from build123d import *

# Parameters (mm, degrees)
SKETCH_1_R          = 36.5
SKETCH_1_R_2        = 28
EXTRUDE_1_DEPTH     = 5.5
SKETCH_2_R          = 31.1
CUT_EXTRUDE_1_DEPTH = 3.3
CUT_EXTRUDE_2_REACH = 53.911
SKETCH_3_R          = 1.55
SKETCH_4_R          = 1.55
CUT_EXTRUDE_3_DEPTH = 3.2


with BuildPart() as part:
    # 草图1 → 凸台-拉伸1 (new body)
    with BuildSketch(Plane(origin=(0, 0, 0), x_dir=(0, 0, -1), z_dir=(1, 0, 0))):
        Circle(SKETCH_1_R)
        Circle(SKETCH_1_R_2, mode=Mode.SUBTRACT)
    extrude(amount=EXTRUDE_1_DEPTH)

    # 草图2 → 切除-拉伸1 (cut)
    with BuildSketch(Plane.ZY):
        Circle(SKETCH_2_R)
    extrude(amount=-CUT_EXTRUDE_1_DEPTH, mode=Mode.SUBTRACT)

    # 草图3 → 切除-拉伸2 (cut, up to next)
    with BuildSketch(Plane(origin=(5.5, 0, 0), x_dir=(0, 0, -1), z_dir=(1, 0, 0)), mode=Mode.PRIVATE) as cut_extrude_2_sk1:
        with Locations((32.9, 0)):
            Circle(SKETCH_3_R)
    cut_extrude_2_tool1 = extrude(cut_extrude_2_sk1.sketch, amount=-CUT_EXTRUDE_2_REACH, mode=Mode.PRIVATE) & part.part
    # 草图3 → 切除-拉伸2 (cut, up to next)
    with BuildSketch(Plane(origin=(5.5, 0, 0), x_dir=(0, 0, -1), z_dir=(1, 0, 0)), mode=Mode.PRIVATE) as cut_extrude_2_sk2:
        with Locations((23.263813101, -23.263813101)):
            Circle(SKETCH_3_R)
    cut_extrude_2_tool2 = extrude(cut_extrude_2_sk2.sketch, amount=-CUT_EXTRUDE_2_REACH, mode=Mode.PRIVATE) & part.part
    # 草图3 → 切除-拉伸2 (cut, up to next)
    with BuildSketch(Plane(origin=(5.5, 0, 0), x_dir=(0, 0, -1), z_dir=(1, 0, 0)), mode=Mode.PRIVATE) as cut_extrude_2_sk3:
        with Locations((0, -32.9)):
            Circle(SKETCH_3_R)
    cut_extrude_2_tool3 = extrude(cut_extrude_2_sk3.sketch, amount=-CUT_EXTRUDE_2_REACH, mode=Mode.PRIVATE) & part.part
    # 草图3 → 切除-拉伸2 (cut, up to next)
    with BuildSketch(Plane(origin=(5.5, 0, 0), x_dir=(0, 0, -1), z_dir=(1, 0, 0)), mode=Mode.PRIVATE) as cut_extrude_2_sk4:
        with Locations((-23.263813101, -23.263813101)):
            Circle(SKETCH_3_R)
    cut_extrude_2_tool4 = extrude(cut_extrude_2_sk4.sketch, amount=-CUT_EXTRUDE_2_REACH, mode=Mode.PRIVATE) & part.part
    # 草图3 → 切除-拉伸2 (cut, up to next)
    with BuildSketch(Plane(origin=(5.5, 0, 0), x_dir=(0, 0, -1), z_dir=(1, 0, 0)), mode=Mode.PRIVATE) as cut_extrude_2_sk5:
        with Locations((-32.9, 0)):
            Circle(SKETCH_3_R)
    cut_extrude_2_tool5 = extrude(cut_extrude_2_sk5.sketch, amount=-CUT_EXTRUDE_2_REACH, mode=Mode.PRIVATE) & part.part
    # 草图3 → 切除-拉伸2 (cut, up to next)
    with BuildSketch(Plane(origin=(5.5, 0, 0), x_dir=(0, 0, -1), z_dir=(1, 0, 0)), mode=Mode.PRIVATE) as cut_extrude_2_sk6:
        with Locations((-23.263813101, 23.263813101)):
            Circle(SKETCH_3_R)
    cut_extrude_2_tool6 = extrude(cut_extrude_2_sk6.sketch, amount=-CUT_EXTRUDE_2_REACH, mode=Mode.PRIVATE) & part.part
    # 草图3 → 切除-拉伸2 (cut, up to next)
    with BuildSketch(Plane(origin=(5.5, 0, 0), x_dir=(0, 0, -1), z_dir=(1, 0, 0)), mode=Mode.PRIVATE) as cut_extrude_2_sk7:
        with Locations((0, 32.9)):
            Circle(SKETCH_3_R)
    cut_extrude_2_tool7 = extrude(cut_extrude_2_sk7.sketch, amount=-CUT_EXTRUDE_2_REACH, mode=Mode.PRIVATE) & part.part
    # 草图3 → 切除-拉伸2 (cut, up to next)
    with BuildSketch(Plane(origin=(5.5, 0, 0), x_dir=(0, 0, -1), z_dir=(1, 0, 0)), mode=Mode.PRIVATE) as cut_extrude_2_sk8:
        with Locations((23.263813101, 23.263813101)):
            Circle(SKETCH_3_R)
    cut_extrude_2_tool8 = extrude(cut_extrude_2_sk8.sketch, amount=-CUT_EXTRUDE_2_REACH, mode=Mode.PRIVATE) & part.part
    add(cut_extrude_2_tool1.solids().sort_by_distance((5.5, 0, -32.9))[0], mode=Mode.SUBTRACT)
    add(cut_extrude_2_tool2.solids().sort_by_distance((5.5, -23.263813, -23.263813))[0], mode=Mode.SUBTRACT)
    add(cut_extrude_2_tool3.solids().sort_by_distance((5.5, -32.9, 0))[0], mode=Mode.SUBTRACT)
    add(cut_extrude_2_tool4.solids().sort_by_distance((5.5, -23.263813, 23.263813))[0], mode=Mode.SUBTRACT)
    add(cut_extrude_2_tool5.solids().sort_by_distance((5.5, 0, 32.9))[0], mode=Mode.SUBTRACT)
    add(cut_extrude_2_tool6.solids().sort_by_distance((5.5, 23.263813, 23.263813))[0], mode=Mode.SUBTRACT)
    add(cut_extrude_2_tool7.solids().sort_by_distance((5.5, 32.9, 0))[0], mode=Mode.SUBTRACT)
    add(cut_extrude_2_tool8.solids().sort_by_distance((5.5, 23.263813, -23.263813))[0], mode=Mode.SUBTRACT)

    # 草图4 → 切除-拉伸3 (cut)
    # profile 1 of 8: a face of its own
    with BuildSketch(Plane(origin=(5.5, 0, 0), x_dir=(0, 0, -1), z_dir=(1, 0, 0))):
        with BuildLine():
            Line((-32.656757596, 2.889780811), (-36.359328813, 3.20143847))
            ThreePointArc((-36.359328813, 3.20143847), (-36.5, 0), (-36.359328813, -3.20143847))
            Line((-36.359328813, -3.20143847), (-32.656757596, -2.889780811))
            ThreePointArc((-32.656757596, -2.889780811), (-30, 0), (-32.656757596, 2.889780811))
        make_face()
        with Locations((-32.9, 0)):
            Circle(SKETCH_4_R, mode=Mode.SUBTRACT)
    # profile 2 of 8: a face of its own
    with BuildSketch(Plane(origin=(5.5, 0, 0), x_dir=(0, 0, -1), z_dir=(1, 0, 0))):
        with BuildLine():
            Line((2.889780811, 32.656757596), (3.20143847, 36.359328813))
            ThreePointArc((3.20143847, 36.359328813), (0, 36.5), (-3.20143847, 36.359328813))
            Line((-3.20143847, 36.359328813), (-2.889780811, 32.656757596))
            ThreePointArc((-2.889780811, 32.656757596), (0, 30), (2.889780811, 32.656757596))
        make_face()
        with Locations((0, 32.9)):
            Circle(SKETCH_4_R, mode=Mode.SUBTRACT)
    # profile 3 of 8: a face of its own
    with BuildSketch(Plane(origin=(5.5, 0, 0), x_dir=(0, 0, -1), z_dir=(1, 0, 0))):
        Polygon((26.498342809, 24.130502724), (24.130502724, 26.498342809), (20.895973016, 25.631653186), (20.029283393, 22.397123478), (22.397123478, 20.029283393), (25.631653186, 20.895973016), align=None)
        with Locations((23.263813101, 23.263813101)):
            Circle(SKETCH_4_R, mode=Mode.SUBTRACT)
    # profile 4 of 8: a face of its own
    with BuildSketch(Plane(origin=(5.5, 0, 0), x_dir=(0, 0, -1), z_dir=(1, 0, 0))):
        with BuildLine():
            Line((36.359328813, 3.20143847), (32.656757596, 2.889780811))
            ThreePointArc((32.656757596, 2.889780811), (30, 0), (32.656757596, -2.889780811))
            Line((32.656757596, -2.889780811), (36.359328813, -3.20143847))
            ThreePointArc((36.359328813, -3.20143847), (36.464815245, -1.602263763), (36.5, 0))
            ThreePointArc((36.5, 0), (36.464815245, 1.602263763), (36.359328813, 3.20143847))
        make_face()
        with Locations((32.9, 0)):
            Circle(SKETCH_4_R, mode=Mode.SUBTRACT)
    # profile 5 of 8: a face of its own
    with BuildSketch(Plane(origin=(5.5, 0, 0), x_dir=(0, 0, -1), z_dir=(1, 0, 0))):
        Polygon((24.130502724, -26.498342809), (26.498342809, -24.130502724), (25.631653186, -20.895973016), (22.397123478, -20.029283393), (20.029283393, -22.397123478), (20.895973016, -25.631653186), align=None)
        with Locations((23.263813101, -23.263813101)):
            Circle(SKETCH_4_R, mode=Mode.SUBTRACT)
    # profile 6 of 8: a face of its own
    with BuildSketch(Plane(origin=(5.5, 0, 0), x_dir=(0, 0, -1), z_dir=(1, 0, 0))):
        with BuildLine():
            ThreePointArc((-3.20143847, -36.359328813), (0, -36.5), (3.20143847, -36.359328813))
            Line((3.20143847, -36.359328813), (2.889780811, -32.656757596))
            ThreePointArc((2.889780811, -32.656757596), (0, -30), (-2.889780811, -32.656757596))
            Line((-2.889780811, -32.656757596), (-3.20143847, -36.359328813))
        make_face()
        with Locations((0, -32.9)):
            Circle(SKETCH_4_R, mode=Mode.SUBTRACT)
    # profile 7 of 8: a face of its own
    with BuildSketch(Plane(origin=(5.5, 0, 0), x_dir=(0, 0, -1), z_dir=(1, 0, 0))):
        Polygon((-20.895973016, -25.631653186), (-20.029283393, -22.397123478), (-22.397123478, -20.029283393), (-25.631653186, -20.895973016), (-26.498342809, -24.130502724), (-24.130502724, -26.498342809), align=None)
    # profile 8 of 8: a face of its own
    with BuildSketch(Plane(origin=(5.5, 0, 0), x_dir=(0, 0, -1), z_dir=(1, 0, 0))):
        Polygon((-20.029283393, 22.397123478), (-20.895973016, 25.631653186), (-24.130502724, 26.498342809), (-26.498342809, 24.130502724), (-25.631653186, 20.895973016), (-22.397123478, 20.029283393), align=None)
    extrude(amount=-CUT_EXTRUDE_3_DEPTH, mode=Mode.SUBTRACT)


solid = part.part
Check sheet for the modelled part. Datum: model origin and axes. Units: mm. A direction names the side the tool comes from. Give positions to 0.01 mm unless a question says otherwise; leave off trailing zeros. Write each loop counter-clockwise with the first axis right and the second up, starting at its lowest first coordinate (ties: lowest second). Pieces come first, ordered by that corner, then holes. Notation, with made-up numbers: (31.5, -12) -> (57.5, -12) arc R17 cw to (57.5, 7) -> close; hole circle Ø8 at (53, 35). An arc over 180 degrees is marked (long way). Use one line per item in the form item = value. Start each with the question number.
1. Section check D-D (y = -8). Record the cut outline in (x, z), and give its area (3 significant figures).
2. Section check A-A (y = 0). Record the cut outline in (x, z).
3. Access from +Z, -Z, +X, -X, +Y, -Y to the whole of each face (thin tool, end or side, straight path). Record for faces 1 (the flat face through (3.922, -34.534, -3.048)), 2 (the flat face through (4.415, 21.23, -21.197)), 3 (the flat face through (2.3, -25, 24)).
4. Mould release check, pull along Y, two halves, no side actions. Record for faces 4 (the cylindrical face through (1.166, -34.413, 0.336)), 5 (the cylindrical face through (4, -30, 0)), 6 (the flat face through (3.922, 34.482, -3.043)): pulls with the +Y half, pulls with the -Y half, needs draft (parallel to the pull), parting line crosses it, or undercut.
5. Section check C-C (z = 17). Record the cut outline in (x, y).
6. Go/stop test with flat-tipped pins: P1, Ø5, axis at y = 25, z = -22, coming from the +X side; P2, Ø3, axis at y = -24.5, z = -23, coming from the +X side; P3, Ø1, axis at x = 1, z = 22.5, coming from the +Y side; P4, Ø1, axis at x = 1, z = -19.5, coming from the +Y side. Record where each tip stops, or that it passes through.
7. Thickness scan on line 1 along Y through (x, z) = (0.7, 0); line 2 along Z through (x, y) = (2.9, -17.5); line 3 along Y through (x, z) = (1.35, 26). Record the ranges inside material, lowest first. Write a range as from..to.
Conclusion:
q1.outline = (0, -35.61) -> (5.5, -35.61) -> (5.5, -26.83) -> (3.3, -26.83) -> (3.3, -30.05) -> (0, -30.05) -> close; (0, 30.05) -> (3.3, 30.05) -> (3.3, 26.83) -> (5.5, 26.83) -> (5.5, 35.61) -> (0, 35.61) -> close
q1.area = 75.3 mm²
q2.outline = (0, -36.5) -> (2.3, -36.5) -> (2.3, -34.45) -> (0, -34.45) -> close; (0, -31.35) -> (2.3, -31.35) -> (2.3, -31.1) -> (0, -31.1) -> close; (0, 31.1) -> (2.3, 31.1) -> (2.3, 31.35) -> (0, 31.35) -> close; (0, 34.45) -> (2.3, 34.45) -> (2.3, 36.5) -> (0, 36.5) -> close; (3.3, -30) -> (5.5, -30) -> (5.5, -28) -> (3.3, -28) -> close; (3.3, 28) -> (5.5, 28) -> (5.5, 30) -> (3.3, 30) -> close
q3.face_1 = +X, -Y
q3.face_2 = +X, -X
q3.face_3 = +X
q4.face_4 = undercut
q4.face_5 = pulls with the -Y half
q4.face_6 = pulls with the +Y half
q5.outline = (0, -32.3) -> (5.5, -32.3) -> (5.5, -22.25) -> (3.3, -22.25) -> (3.3, -26.04) -> (0, -26.04) -> close; (0, 26.04) -> (3.3, 26.04) -> (3.3, 22.25) -> (5.5, 22.25) -> (5.5, 32.3) -> (0, 32.3) -> close
q6.P1 = 5.5
q6.P2 = 2.3
q6.P3 = 29.12
q6.P4 = 31.16
q7.line_1 = -36.5..-34.45, -31.35..-31.1, 31.1..31.35, 34.45..36.5
q7.line_2 = -32.03..-25.71, 25.71..32.03
q7.line_3 = -25.62..-17.06, 17.06..25.62
